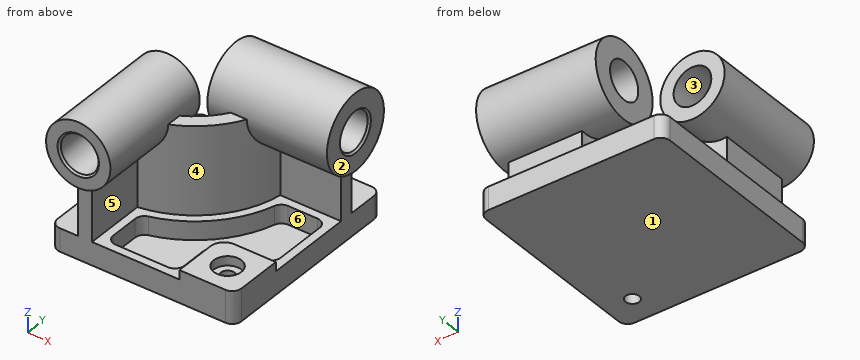
from build123d import *

# Parameters (mm, degrees)
SKETCH1_W                               = 200
SKETCH1_H                               = 213
BOSS_EXTRUDE1_DEPTH                     = 25
BOSS_EXTRUDE2_DEPTH                     = 10
FILLET1_R                               = 10
EXTRUDE_THIN1_DEPTH                     = 95
BOSS_EXTRUDE3_DEPTH                     = 10
BOSS_EXTRUDE3_DEPTH_BACK                = 120
SKETCH5_R                               = 35
BOSS_EXTRUDE4_DEPTH                     = 10
BOSS_EXTRUDE4_DEPTH_BACK                = 120
SKETCH6_R                               = 41.5
CUT_EXTRUDE1_REACH                      = 298.498
SKETCH7_R                               = 20.5
CUT_EXTRUDE2_REACH                      = 291.404
SKETCH8_R                               = 20.5
CHAMFER1_SIZE                           = 2
CUT_EXTRUDE3_DEPTH                      = 20
CBORE_FOR_M8_HEX_HEAD_BOLT1_D           = 15
CBORE_FOR_M8_HEX_HEAD_BOLT1_CBORE_D     = 30
CBORE_FOR_M8_HEX_HEAD_BOLT1_CBORE_DEPTH = 10


with BuildPart() as part:
    # Sketch1 → Boss-Extrude1 (new body)
    with BuildSketch(Plane.XY):
        Rectangle(SKETCH1_W, SKETCH1_H)
    extrude(amount=BOSS_EXTRUDE1_DEPTH)

    # Sketch3 → Boss-Extrude2 (add)
    with BuildSketch(Plane.XY.offset(25)):
        with BuildLine():
            Line((100, -106.5), (40, -106.5))
            Line((40, -106.5), (40, -61.5))
            ThreePointArc((40, -61.5), (44.393398282, -50.893398282), (55, -46.5))
            Line((55, -46.5), (100, -46.5))
            Line((100, -46.5), (100, -106.5))
        make_face()
    extrude(amount=BOSS_EXTRUDE2_DEPTH)

    # Fillet1
    fillet1_edges = [part.edges().sort_by_distance(p)[0] for p in [
        (100, -106.5, 17.5),
        (-100, -106.5, 12.5),
        (-100, 106.5, 12.5),
        (100, 106.5, 12.5),
    ]]
    fillet(fillet1_edges, radius=FILLET1_R)

    # Sketch4 → Extrude-Thin1 (add)
    with BuildSketch(Plane.XY.offset(25)):
        with BuildLine():
            Line((100, 63.5), (20, 63.5))
            ThreePointArc((20, 63.5), (-6.360389693, -0.139610307), (-70, -26.5))
            Line((-70, -26.5), (-70, -106.5))
            Line((-70, -106.5), (-60, -106.5))
            Line((-60, -106.5), (-60, -35.998743711))
            ThreePointArc((-60, -35.998743711), (0.710678119, -7.210678119), (29.498743711, 53.5))
            Line((29.498743711, 53.5), (100, 53.5))
            Line((100, 53.5), (100, 63.5))
        make_face()
        with BuildLine():
            Line((-55, -106.5), (-55, -40.423048454))
            ThreePointArc((-55, -40.423048454), (4.246212025, -10.746212025), (33.923048454, 48.5))
            Line((33.923048454, 48.5), (100, 48.5))
            Line((100, 48.5), (100, 58.5))
            Line((100, 58.5), (24.868329805, 58.5))
            ThreePointArc((24.868329805, 58.5), (-2.824855787, -3.675144213), (-65, -31.368329805))
            Line((-65, -31.368329805), (-65, -106.5))
            Line((-65, -106.5), (-55, -106.5))
        make_face()
    extrude(amount=EXTRUDE_THIN1_DEPTH)

    # Sketch5 → Boss-Extrude3 (add, two sides: drawn at the far end of the back side and taken through both)
    with BuildSketch(Plane.XZ.offset(106.5).offset(-BOSS_EXTRUDE3_DEPTH_BACK)):
        with Locations(Location((-62.5, 120, 0), (0, 0, 270))):
            Circle(SKETCH5_R)
    extrude(amount=BOSS_EXTRUDE3_DEPTH + BOSS_EXTRUDE3_DEPTH_BACK)

    # Sketch6 → Boss-Extrude4 (add, two sides: drawn at the far end of the back side and taken through both)
    with BuildSketch(Plane(origin=(100, 0, 0), x_dir=(0, 0, -1), z_dir=(1, 0, 0)).offset(-BOSS_EXTRUDE4_DEPTH_BACK)):
        with Locations(Location((-120, 56, 0), (0, 0, 90))):
            Circle(SKETCH6_R)
    extrude(amount=BOSS_EXTRUDE4_DEPTH + BOSS_EXTRUDE4_DEPTH_BACK)

    # Sketch7 → Cut-Extrude1 (cut, up to next)
    with BuildSketch(Plane.XZ.offset(116.5), mode=Mode.PRIVATE) as cut_extrude1_sk1:
        with Locations(Location((-62.5, 120, 0), (0, 0, 270))):
            Circle(SKETCH7_R)
    cut_extrude1_tool1 = extrude(cut_extrude1_sk1.sketch, amount=-CUT_EXTRUDE1_REACH, mode=Mode.PRIVATE) & part.part
    add(cut_extrude1_tool1.solids().sort_by_distance((-62.5, -116.5, 120))[0], mode=Mode.SUBTRACT)

    # Sketch8 → Cut-Extrude2 (cut, up to next)
    with BuildSketch(Plane(origin=(110, 0, 0), x_dir=(0, 0, -1), z_dir=(1, 0, 0)), mode=Mode.PRIVATE) as cut_extrude2_sk1:
        with Locations(Location((-120, 56, 0), (0, 0, 90))):
            Circle(SKETCH8_R)
    cut_extrude2_tool1 = extrude(cut_extrude2_sk1.sketch, amount=-CUT_EXTRUDE2_REACH, mode=Mode.PRIVATE) & part.part
    add(cut_extrude2_tool1.solids().sort_by_distance((110, 56, 120))[0], mode=Mode.SUBTRACT)

    # Chamfer1
    chamfer1_edges = [part.edges().sort_by_distance(p)[0] for p in [
        (-62.5, -116.5, 140.5),
        (110, 35.5, 120),
    ]]
    chamfer(chamfer1_edges, length=CHAMFER1_SIZE)

    # Sketch9 → Cut-Extrude3 (cut)
    with BuildSketch(Plane.XY.offset(25)):
        with BuildLine():
            Line((-46, -55.747641486), (-46, -87.5))
            ThreePointArc((-46, -87.5), (-43.071067812, -94.571067812), (-36, -97.5))
            Line((-36, -97.5), (21, -97.5))
            ThreePointArc((21, -97.5), (28.071067812, -94.571067812), (31, -87.5))
            Line((31, -87.5), (31, -61.5))
            ThreePointArc((31, -61.5), (38.029437252, -44.529437252), (55, -37.5))
            Line((55, -37.5), (81, -37.5))
            ThreePointArc((81, -37.5), (88.071067812, -34.571067812), (91, -27.5))
            Line((91, -27.5), (91, 29.5))
            ThreePointArc((91, 29.5), (88.071067812, 36.571067812), (81, 39.5))
            Line((81, 39.5), (49.247641486, 39.5))
            ThreePointArc((49.247641486, 39.5), (43.223496519, 37.481834214), (39.630896205, 32.241935484))
            ThreePointArc((39.630896205, 32.241935484), (10.610173055, -17.110173055), (-38.741935484, -46.130896205))
            ThreePointArc((-38.741935484, -46.130896205), (-43.981834214, -49.723496519), (-46, -55.747641486))
        make_face()
    extrude(amount=-CUT_EXTRUDE3_DEPTH, mode=Mode.SUBTRACT)

    # CBORE for M8 Hex Head Bolt1 (through all)
    with Locations(Plane.XY.offset(35)):
        with Locations((70, -76.5)):
            CounterBoreHole(CBORE_FOR_M8_HEX_HEAD_BOLT1_D / 2, CBORE_FOR_M8_HEX_HEAD_BOLT1_CBORE_D / 2, CBORE_FOR_M8_HEX_HEAD_BOLT1_CBORE_DEPTH)


solid = part.part
For this review, take the finished solid that the model builds, in its own axes (mm). Face numbers are marked on the shaded views. A direction names the side the tool comes from. Coordinates: 2 decimals unless noted, no trailing zeros. Loops run counter-clockwise (first coordinate to the right, second up) from the corner with the lowest first, then second, coordinate; pieces in that order, holes last. Notation, with made-up numbers: (-7, 72) - (47, 72) arc R12 ccw to (47, 95) - close; hole circle Ø8 at (19.5, 29). An arc over 180 degrees is marked (long way). Use a Markdown table: item, result. Add a question column.
Item 1: We need section B-B (x = 70). Give the boundary of the cut face in (y, z).
Item 2: Insertion check: pin 1 Ø5 at (x, y) = (22.5, 59) entering from +Z; pin 2 Ø4 at (x, z) = (81, 123) entering from +Y; pin 3 Ø4 at (y, z) = (-93.5, 143.5) entering from -X. Each pin has a flat end and moves straight along its axis. Give the tip position at first contact, or say it passes through.
Item 3: We need section C-C (z = 46). Give the boundary of the cut face in (x, y).
Item 4: For line 1 (X direction, y = -76, z = 9); line 2 (Z direction, x = 33, y = 56); line 3 (Z direction, x = -62, y = -27), list the stretches that pass through material, from the lowest coordinate up.
Item 5: Mouldability with a two-part tool opening along X and no side actions: class the marked faces 1, 2 and 3 as pulls with the +X half, pulls with the -X half, needs draft (parallel to the pull), parting line crosses it, or undercut.
Item 6: We need section A-A (y = -76.5). Give the boundary of the cut face in (x, z), and give its area (3 significant figures).
Item 7: Tool access review of the marked faces 4, 5 and 6: name each direction out of +Z, -Z, +X, -X, +Y, -Y from which nothing blocks a thin tool from reaching the whole face with its end or side.
Item 8: We need section D-D (z = 150.5). Give the boundary of the cut face in (x, y).
Results list:
| question | item | result |
|---|---|---|
| 1 | outline | (-106.5, 0) - (-84, 0) - (-84, 25) - (-91.5, 25) - (-91.5, 35) - (-106.5, 35) - close; (-69, 0) - (106.5, 0) - (106.5, 25) - (63.5, 25) - (63.5, 79.18) arc R41.5 ccw (long way) to (48.5, 79.18) - (48.5, 25) - (39.5, 25) - (39.5, 5) - (-37.5, 5) - (-37.5, 25) - (-46.5, 25) - (-46.5, 35) - (-61.5, 35) - (-61.5, 25) - (-69, 25) - close; hole circle Ø41 at (56, 120) |
| 2 | pin 1 | stops at z = 161.5 |
| 2 | pin 2 | stops at y = 97.49 |
| 2 | pin 3 | stops at x = -90.12 |
| 3 | outline | (-70, -106.5) - (-55, -106.5) - (-55, -40.42) arc R105 ccw to (33.92, 48.5) - (100, 48.5) - (100, 63.5) - (20, 63.5) arc R90 cw to (-70, -26.5) - close |
| 4 | line 1 | x = -100 to -46, 31 to 62.52, 77.48 to 100 |
| 4 | line 2 | z = 0 to 99.5, 140.5 to 161.5 |
| 4 | line 3 | z = 0 to 99.51, 140.49 to 155 |
| 5 | face 1 | needs draft |
| 5 | face 2 | pulls with the +X half |
| 5 | face 3 | undercut |
| 6 | outline | (-100, 0) - (62.5, 0) - (62.5, 25) - (55, 25) - (55, 35) - (40, 35) - (40, 25) - (31, 25) - (31, 5) - (-46, 5) - (-46, 25) - (-55, 25) - (-55, 85.81) arc R35 ccw (long way) to (-70, 85.81) - (-70, 25) - (-100, 25) - close; (77.5, 0) - (100, 0) - (100, 35) - (85, 35) - (85, 25) - (77.5, 25) - close; hole circle Ø41 at (-62.5, 120) |
| 6 | area | 6,820 mm^2 |
| 7 | face 4 | +X, -Y |
| 7 | face 5 | -Y |
| 7 | face 6 | none |
| 8 | outline | (-79.67, -116.5) - (-45.33, -116.5) - (-45.33, 13.5) - (-79.67, 13.5) - close; (-20, 27.86) - (110, 27.86) - (110, 84.14) - (-20, 84.14) - close |
